```python
from build123d import *

# Parameters (mm, degrees)
BOSS_EXTRUDE1_DEPTH = 2.6
BOSS_EXTRUDE2_START = 0.4
SKETCH2_R           = 11
BOSS_EXTRUDE2_DEPTH = 0.4
SKETCH3_R           = 10
BOSS_EXTRUDE3_DEPTH = 5


with BuildPart() as part:
    # Sketch1 → Boss-Extrude1 (new body)
    with BuildSketch(Plane.XY):
        Polygon((-101.82751654, -139.254588807), (-109.82751654, -139.254588807), (-112.82751654, -142.254588807), (-112.82751654, -160.410438888), (-109.82751654, -163.410438888), (-101.82751654, -163.410438888), (-93.82751654, -163.410438888), (-90.82751654, -160.410438888), (-90.82751654, -142.254588807), (-93.82751654, -139.254588807), align=None)
        with BuildLine():
            Line((-101.82751654, -161.410438888), (-101.82751654, -161.406823358))
            add(Edge.make_bspline(
                [(-101.82751654, -161.406823358), (-102.422162271, -161.406823358), (-103.006870259, -161.348469799), (-103.869635205, -161.176988515), (-104.154822959, -161.1057322), (-104.720287744, -160.934384241), (-105.001330007, -160.833809548), (-105.818842439, -160.494941156), (-106.33582072, -160.218450477), (-107.314217622, -159.565215144), (-107.777447082, -159.184998049), (-108.607719596, -158.354451471), (-108.980275796, -157.901273798), (-109.473711648, -157.16329018), (-109.626905607, -156.907604181), (-109.904538968, -156.387928298), (-110.155344462, -155.857224862), (-110.353303759, -155.304799077), (-110.524479072, -154.741363777), (-110.596954867, -154.452589203), (-110.770224625, -153.581187835), (-110.827307979, -152.997176095), (-110.827619973, -152.116665053), (-110.813402769, -151.822407076), (-110.755453282, -151.232336564), (-110.711753861, -150.938362019), (-110.539397258, -150.07260899), (-110.369409104, -149.511563453), (-110.031331697, -148.69431731), (-109.903855236, -148.424565494), (-109.625080406, -147.903123691), (-109.473781689, -147.650944456), (-108.985007402, -146.919418072), (-108.612994329, -146.464837975), (-107.773025896, -145.624478569), (-107.317394389, -145.251329051), (-106.586246745, -144.762472579), (-106.334327243, -144.611225122), (-105.813734345, -144.33263421), (-105.543874944, -144.204932828), (-104.725722152, -143.866107062), (-104.164612328, -143.6960009), (-103.011425471, -143.465984444), (-102.414902795, -143.407128867), (-101.82751654, -143.407128867)],
                knots=[0, 0, 0, 0, 0.0625, 0.0625, 0.09375, 0.09375, 0.125, 0.125, 0.1875, 0.1875, 0.25, 0.25, 0.3125, 0.3125, 0.34375, 0.34375, 0.375, 0.40625, 0.40625, 0.4375, 0.4375, 0.5, 0.5, 0.53125, 0.53125, 0.5625, 0.5625, 0.625, 0.625, 0.65625, 0.65625, 0.6875, 0.6875, 0.75, 0.75, 0.8125, 0.8125, 0.84375, 0.84375, 0.875, 0.875, 0.9375, 0.9375, 1, 1, 1, 1], degree=3))
            Line((-101.82751654, -143.407128867), (-101.82751654, -143.410438888))
            ThreePointArc((-101.82751654, -143.410438888), (-92.82751654, -152.410438888), (-101.82751654, -161.410438888))
        make_face(mode=Mode.SUBTRACT)
    extrude(amount=BOSS_EXTRUDE1_DEPTH)

    # Sketch2 → Boss-Extrude2 (add)
    with BuildSketch(Plane(origin=(0, 0, 3), x_dir=(-1, 0, 0), z_dir=(0, 0, -1)).offset(BOSS_EXTRUDE2_START)):
        with Locations(Location((101.82751654, -152.410438888, 0), (0, 0, 270))):
            Circle(SKETCH2_R)
        with BuildLine():
            Line((101.82751654, -161.410438888), (101.82751654, -161.406823358))
            add(Edge.make_bspline(
                [(101.82751654, -161.406823358), (102.422162271, -161.406823358), (103.006870259, -161.348469799), (103.869635205, -161.176988515), (104.154822959, -161.1057322), (104.720287744, -160.934384241), (105.001330007, -160.833809548), (105.818842439, -160.494941156), (106.33582072, -160.218450477), (107.314217622, -159.565215144), (107.777447082, -159.184998049), (108.607719596, -158.354451471), (108.980275796, -157.901273798), (109.473711648, -157.16329018), (109.626905607, -156.907604181), (109.904538968, -156.387928298), (110.155344462, -155.857224862), (110.353303759, -155.304799077), (110.524479072, -154.741363777), (110.596954867, -154.452589203), (110.770224625, -153.581187835), (110.827307979, -152.997176095), (110.827619973, -152.116665053), (110.813402769, -151.822407076), (110.755453282, -151.232336564), (110.711753861, -150.938362019), (110.539397258, -150.07260899), (110.369409104, -149.511563453), (110.031331697, -148.69431731), (109.903855236, -148.424565494), (109.625080406, -147.903123691), (109.473781689, -147.650944456), (108.985007402, -146.919418072), (108.612994329, -146.464837975), (107.773025896, -145.624478569), (107.317394389, -145.251329051), (106.586246745, -144.762472579), (106.334327243, -144.611225122), (105.813734345, -144.33263421), (105.543874944, -144.204932828), (104.725722152, -143.866107062), (104.164612328, -143.6960009), (103.011425471, -143.465984444), (102.414902795, -143.407128867), (101.82751654, -143.407128867)],
                knots=[0, 0, 0, 0, 0.0625, 0.0625, 0.09375, 0.09375, 0.125, 0.125, 0.1875, 0.1875, 0.25, 0.25, 0.3125, 0.3125, 0.34375, 0.34375, 0.375, 0.40625, 0.40625, 0.4375, 0.4375, 0.5, 0.5, 0.53125, 0.53125, 0.5625, 0.5625, 0.625, 0.625, 0.65625, 0.65625, 0.6875, 0.6875, 0.75, 0.75, 0.8125, 0.8125, 0.84375, 0.84375, 0.875, 0.875, 0.9375, 0.9375, 1, 1, 1, 1], degree=3))
            Line((101.82751654, -143.407128867), (101.82751654, -143.410438888))
            ThreePointArc((101.82751654, -143.410438888), (92.82751654, -152.410438888), (101.82751654, -161.410438888))
        make_face(mode=Mode.SUBTRACT)
    extrude(amount=-BOSS_EXTRUDE2_DEPTH)

    # Sketch3 → Boss-Extrude3 (add)
    with BuildSketch(Plane.XY.offset(3)):
        with Locations(Location((-101.82751654, -152.410438888, 0), (0, 0, 180))):
            Circle(SKETCH3_R)
        with BuildLine():
            Line((-101.82751654, -161.406823358), (-101.82751654, -161.410438888))
            ThreePointArc((-101.82751654, -161.410438888), (-92.82751654, -152.410438888), (-101.82751654, -143.410438888))
            Line((-101.82751654, -143.410438888), (-101.82751654, -143.407128867))
            add(Edge.make_bspline(
                [(-101.82751654, -143.407128867), (-102.414902795, -143.407128867), (-103.011425471, -143.465984444), (-104.164612328, -143.6960009), (-104.725722152, -143.866107062), (-105.543874944, -144.204932828), (-105.813734345, -144.33263421), (-106.334327243, -144.611225122), (-106.586246745, -144.762472579), (-107.317394389, -145.251329051), (-107.773025896, -145.624478569), (-108.612994329, -146.464837975), (-108.985007402, -146.919418072), (-109.473781689, -147.650944456), (-109.625080406, -147.903123691), (-109.903855236, -148.424565494), (-110.031331697, -148.69431731), (-110.369409104, -149.511563453), (-110.539397258, -150.07260899), (-110.711753861, -150.938362019), (-110.755453282, -151.232336564), (-110.813402769, -151.822407076), (-110.827619973, -152.116665053), (-110.827307979, -152.997176095), (-110.770224625, -153.581187835), (-110.596954867, -154.452589203), (-110.524479072, -154.741363777), (-110.353303759, -155.304799077), (-110.155344462, -155.857224862), (-109.904538968, -156.387928298), (-109.626905607, -156.907604181), (-109.473711648, -157.16329018), (-108.980275796, -157.901273798), (-108.607719596, -158.354451471), (-107.777447082, -159.184998049), (-107.314217622, -159.565215144), (-106.33582072, -160.218450477), (-105.818842439, -160.494941156), (-105.001330007, -160.833809548), (-104.720287744, -160.934384241), (-104.154822959, -161.1057322), (-103.869635205, -161.176988515), (-103.006870259, -161.348469799), (-102.422162271, -161.406823358), (-101.82751654, -161.406823358)],
                knots=[0, 0, 0, 0, 0.0625, 0.0625, 0.125, 0.125, 0.15625, 0.15625, 0.1875, 0.1875, 0.25, 0.25, 0.3125, 0.3125, 0.34375, 0.34375, 0.375, 0.375, 0.4375, 0.4375, 0.46875, 0.46875, 0.5, 0.5, 0.5625, 0.5625, 0.59375, 0.59375, 0.625, 0.65625, 0.65625, 0.6875, 0.6875, 0.75, 0.75, 0.8125, 0.8125, 0.875, 0.875, 0.90625, 0.90625, 0.9375, 0.9375, 1, 1, 1, 1], degree=3))
        make_face(mode=Mode.SUBTRACT)
    extrude(amount=BOSS_EXTRUDE3_DEPTH)


solid = part.part
```
CAD build for the part. Positions are in the model's coordinates, mm. A direction names the side the tool comes from. Coordinates: 2 decimals unless noted, no trailing zeros. Order: outer loops, then holes, each group sorted by start corner. A loop starts at its lowest first (then second) coordinate and runs counter-clockwise, first axis right, second up.
(1) Which spindle directions (+Z, -Z, +X, -X, +Y, -Y) get a long thin tool onto all of the face, cutting with end or side? Do faces 1 (the face through (-111.307, -140.734, 1.282)), 2 (the face through (-110, -161, 2.6)), 3 (the face through (-102, -139.255, 1)), 4 (the face through (-101, -141, 2.6)), 5 (the face through (-92, -155, 3)). Say none if no direction does.
Solution:
face 1: +Z, -Z, -X, +Y
face 2: +Z, -X, -Y
face 3: +Z, -Z, +X, -X, +Y
face 4: +Z, +Y
face 5: +Z
(2) Mould opens along X. For faces 6 (the face through (-92.83, -152.61, 3.94)), 7 (the face through (-111.103, -158.324, 2.797)), 8 (the face through (-90.828, -151, 1)), 9 (the face through (-93.5, -160.3, 2.6)) say: released by +X, released by -X, zero draft, split by the parting line, or undercut.
Solution:
face 6: undercut
face 7: split by the parting line
face 8: released by +X
face 9: zero draft
(3) Saw through at C-C, the plane x = -92.25. Write the cut outline in (y, z).
Solution:
outline: (-161.83, 0) - (-140.83, 0) - (-140.83, 2.6) - (-147, 2.6) - (-147, 3) - (-149.53, 3) - (-149.53, 8) - (-155.29, 8) - (-155.29, 3) - (-157.82, 3) - (-157.82, 2.6) - (-161.83, 2.6) - close
(4) Pin check, flat tips, straight feed: pin 1 Ø1.5 at (x, z) = (-100, 6.5) entering from +Y; pin 2 Ø1.5 at (y, z) = (-153.5, 4) entering from -X. Stop position of each tip, or through.
Solution:
pin 1: stops at y = -142.47
pin 2: stops at x = -111.82
(5) Saw through at A-A, the plane x = -98.25. Write the cut outline in (y, z).
Solution:
outline: (-163.41, 0) - (-160.67, 0) - (-160.67, 8) - (-161.75, 8) - (-161.75, 3) - (-162.81, 3) - (-162.81, 2.6) - (-163.41, 2.6) - close; (-144.15, 0) - (-139.25, 0) - (-139.25, 2.6) - (-142.01, 2.6) - (-142.01, 3) - (-143.07, 3) - (-143.07, 8) - (-144.15, 8) - close
(6) Saw through at B-B, the plane x = -94.5. Write the cut outline in (y, z), and give its area (3 significant figures).
Solution:
outline: (-163.41, 0) - (-157.64, 0) - (-157.64, 8) - (-159.22, 8) - (-159.22, 3) - (-160.61, 3) - (-160.61, 2.6) - (-163.41, 2.6) - close; (-147.18, 0) - (-139.25, 0) - (-139.25, 2.6) - (-144.21, 2.6) - (-144.21, 3) - (-145.61, 3) - (-145.61, 8) - (-147.18, 8) - close
area: 53.8 mm2
(7) Drill centre lines: L1, parallel to Y at x = -101.5, z = 4.75; L2, parallel to X at y = -149, z = 7.5; L3, parallel to X at y = -145.25, z = 7. Where is each one in solid material? Low to high.
Solution:
L1: y = -162.41 to -161.4, -143.42 to -142.42
L2: x = -111.23 to -110.16, -93.5 to -92.43
L3: x = -108.81 to -107.28, -96.38 to -94.85
